Here's how the part is built. I have some questions about the finished solid (model axes, mm). A direction names the side the tool comes from. Round coordinates to 2 decimals unless told otherwise and drop trailing zeros. Loops run counter-clockwise (first coordinate to the right, second up) from the corner with the lowest first, then second, coordinate; pieces in that order, holes last. Notation, with made-up numbers: (-11.75, 71) - (11.25, 71) arc R33 ccw to (11.25, 103) - close; hole circle Ø6 at (46.5, 66.5). An arc over 180 degrees is marked (long way). Return JSON: item names as keys, results as strings. Group by question number.
Autodesk Inventor part; units mm, degrees
ref_plane "YZ Plane" through (0, 0, 0) normal (1, 0, 0) x (0, 1, 0)
ref_plane "XZ Plane" through (0, 0, 0) normal (0, 1, 0) x (-1, 0, 0)
ref_plane "XY Plane" through (0, 0, 0) normal (0, 0, 1) x (1, 0, 0)
sketch "Sketch1" plane through (0, 0, 0) normal (0, 1, 0) x (-1, 0, 0)
  circle A0 centre (0, 0) radius 22.5
  line L0 (55, -55) -> (-55, -55)
  line L1 (-55, -55) -> (-55, 55)
  line L2 (-55, 55) -> (55, 55)
  line L3 (55, 55) -> (55, -55)
  line L4 (55, -55) -> (-55, 55) construction
  line L5 (-55, -55) -> (55, 55) construction
  circle A1 centre (0, 0) radius 16.4
  dimension "d0" = 45
  dimension "d1" = 110
  dimension "d2" = 110
  dimension "d3" = 32.8
extrude "Extrusion1" add sketch "Sketch1" along normal blind 6 contours L0 L1 L2 L3
extrude "Extrusion2" add sketch "Sketch1" along normal blind 60 contours A0
chamfer "Chamfer1" distance 10 angle 45 1 edges at (22.5, 6, 0)
sketch "Sketch3" plane through (0, 6, 0) normal (0, 1, 0) x (1, 0, 0)
  line L0 (55, -55) -> (55, 55)
  line L1 (55, 55) -> (-55, 55)
  line L2 (-55, -55) -> (55, -55)
  line L3 (-55, 55) -> (-55, -55)
  point P0 (0, 0)
  point P1 (-45, 45)
  point P2 (-45, -45)
  point P3 (45, -45)
  point P4 (45, 45)
  point P5 (55, 0)
  point P6 (0, 55)
  point P7 (0, -55)
  point P8 (-55, 0)
  dimension "d14" = 10
  dimension "d15" = 10
  dimension "d16" = 10
  dimension "d17" = 10
hole "Hole1" at (-45, 6, -45) at (45, 6, -45) at (45, 6, 45) at (-45, 6, 45) direction (0, -1, 0) diameter 8.5 end through all counterbore diameter 18.01 counterbore depth 2
sketch "Sketch4" plane through (-55, 0, 55) normal (0, 0, 1) x (1, 0, 0)
  line L0 (0, 0) -> (110, 0)
  line L1 (77.5, 60) -> (32.5, 60)
  point P0 (55, 0)
  point P1 (55, 45)
  point P2 (55, 0)
  dimension "d25" = 15
hole "Hole2" at (0, 45, 55) direction (0, 0, -1) diameter 8.5 end through all
chamfer "Chamfer2" distance 10 angle 45 1 edges at (22.5, 16, 0)
chamfer "Chamfer3" distance 5 angle 45 1 edges at (22.5, 26, 0)
properties part number "Soporte_Vertical_Para_Balancin" material "ABS Plastic"
Q1. If we mould it in two halves opening along Z, with no side actions, what happens to faces 1 (the flat face through (1, 3, 55)), 2 (the cylindrical face through (44.813, 1.972, 40.754)), 3 (the cylindrical face through (4.878, 45.297, 21.965)), 4 (the cylindrical face through (-0.187, 49.246, -19.217))? For each: +Z half, -Z half, draft (parallel to the pull), parting line (faces both ways), or undercut.
Q2. Imagine slicing it at C-C, the plane y = 38.5. List the corners of the cut face in (x, z) for me, and give its area (3 significant figures).
Q3. Please list where these lines run through material, in increasing order: line 1 (Z direction, x = -45, y = 1.9); line 2 (Z direction, x = -45, y = 4.95) (3 decimals).
Q4. Will these pins go through, and if not, where does the flat tip stop? pin 1 Ø3 at (x, z) = (-34, -20.5) entering from +Y; pin 2 Ø5.5 at (x, z) = (-41, -46) entering from +Y; pin 3 Ø6 at (x, y) = (-19, 14) entering from +Z.
Q5. Imagine slicing it at D-D, the plane x = 0. Give the number of separate pieces and of enclosed holes in the cut face, and give its area (3 significant figures).
Q6. Imagine slicing it at A-A, the plane z = -45. List the corners of the cut face in (x, y) for me (3 decimals), and give its area (3 significant figures).
Q7. For faces 5 (the cylindrical face through (-42.41, 1.97, 41.63)), 6 (the flat face through (-41, 4, -43)), which set-ups out of +Z, -Z, +X, -X, +Y, -Y let a thin tool reach every point of the face, with its end or its side?
Q8. Imagine slicing it at B-B, the plane y = 47. List the corners of the cut face in (x, z) for me, and give its area (3 significant figures).
Output values:
{
 "1": {"face 1": "+Z half", "face 2": "undercut", "face 3": "parting line", "face 4": "draft"},
 "2": {"outline": "circle Ø45 at (0, 0); hole circle Ø32.8 at (0, 0)", "area": "745 mm^2"},
 "3": {"line 1": "z = -55 to -49.25, -40.75 to 40.75, 49.25 to 55", "line 2": "z = -55 to -54.005, -35.995 to 35.995, 54.005 to 55"},
 "4": {"pin 1": "stops at y = 6", "pin 2": "stops at y = 4", "pin 3": "stops at z = 22.82"},
 "5": {"separate pieces": "4", "enclosed holes": "0", "area": "1,200 mm^2"},
 "6": {"outline": "(-55, 0) - (-49.25, 0) - (-49.25, 4) - (-54.005, 4) - (-54.005, 6) - (-55, 6) - close; (-40.75, 0) - (40.75, 0) - (40.75, 4) - (35.995, 4) - (35.995, 6) - (-35.995, 6) - (-35.995, 4) - (-40.75, 4) - close; (49.25, 0) - (55, 0) - (55, 6) - (54.005, 6) - (54.005, 4) - (49.25, 4) - close", "area": "520 mm^2"},
 "7": {"face 5": "+Y, -Y", "face 6": "+Y"},
 "8": {"outline": "(-3.75, -22.19) - (-3.75, -15.97) arc R16.4 cw to (-3.75, 15.97) - (-3.75, 22.19) arc R22.5 ccw to start; (3.75, -22.19) arc R22.5 ccw to (3.75, 22.19) - (3.75, 15.97) arc R16.4 cw to (3.75, -15.97) - close", "area": "653 mm^2"}
}
